```python
from build123d import *

# Parameters (mm, degrees)
RESSALTO_EXTRUS_O2_DEPTH      = 30
RESSALTO_EXTRUS_O3_DEPTH      = 3
RESSALTO_EXTRUS_O4_DEPTH      = 3
RESSALTO_EXTRUS_O4_DEPTH_BACK = 10


with BuildPart() as part:
    # Esboço2 → Ressalto-extrusão2 (new body)
    with BuildSketch(Plane(origin=(0, 0, 0), x_dir=(0, 0, -1), z_dir=(1, 0, 0))):
        with BuildLine():
            Line((2.90159992, -0.062465938), (-35.09840008, -0.062465938))
            Line((-35.09840008, -0.062465938), (-39.886084903, -0.062465938))
            ThreePointArc((-39.886084903, -0.062465938), (-45.202180234, 1.467638524), (-48.891439328, 5.589707975))
            ThreePointArc((-48.891439328, 5.589707975), (-52.096536948, 9.772081499), (-56.69840008, 12.338743681))
            ThreePointArc((-56.69840008, 12.338743681), (-59.373224015, 11.895603401), (-60.59840008, 9.476926077))
            Line((-60.59840008, 9.476926077), (-60.59840008, 20.976926077))
            ThreePointArc((-60.59840008, 20.976926077), (-59.719720424, 23.09824642), (-57.59840008, 23.976926077))
            Line((-57.59840008, 23.976926077), (25.40159992, 23.976926077))
            ThreePointArc((25.40159992, 23.976926077), (27.522920263, 23.09824642), (28.40159992, 20.976926077))
            Line((28.40159992, 20.976926077), (28.40159992, 9.476926077))
            ThreePointArc((28.40159992, 9.476926077), (27.176423855, 11.895603401), (24.50159992, 12.338743681))
            ThreePointArc((24.50159992, 12.338743681), (19.899736788, 9.772081499), (16.694639168, 5.589707975))
            ThreePointArc((16.694639168, 5.589707975), (13.005380073, 1.467638524), (7.689284743, -0.062465938))
            Line((7.689284743, -0.062465938), (2.90159992, -0.062465938))
        make_face()
    extrude(amount=RESSALTO_EXTRUS_O2_DEPTH)

    # Esboço3 → Ressalto-extrusão3 (add)
    with BuildSketch(Plane.ZY):
        with BuildLine():
            Line((60.59840008, 15.226926077), (60.59840008, 20.976926077))
            ThreePointArc((60.59840008, 20.976926077), (59.719720424, 23.09824642), (57.59840008, 23.976926077))
            Line((57.59840008, 23.976926077), (16.09840008, 23.976926077))
            Line((16.09840008, 23.976926077), (-25.40159992, 23.976926077))
            ThreePointArc((-25.40159992, 23.976926077), (-27.522920263, 23.09824642), (-28.40159992, 20.976926077))
            Line((-28.40159992, 20.976926077), (-28.40159992, 15.226926077))
            Line((-28.40159992, 15.226926077), (-28.40159992, -16.773073923))
            ThreePointArc((-28.40159992, -16.773073923), (-27.522920263, -18.894394267), (-25.40159992, -19.773073923))
            Line((-25.40159992, -19.773073923), (57.59840008, -19.773073923))
            ThreePointArc((57.59840008, -19.773073923), (59.719720424, -18.894394267), (60.59840008, -16.773073923))
            Line((60.59840008, -16.773073923), (60.59840008, 15.226926077))
        make_face()
    extrude(amount=RESSALTO_EXTRUS_O3_DEPTH)

    # Esboço4 → Ressalto-extrusão4 (add, two sides)
    with BuildSketch(Plane(origin=(30, 0, 0), x_dir=(0, 0, -1), z_dir=(1, 0, 0))) as ressalto_extrus_o4_sk:
        with BuildLine():
            Line((-16.09840008, 23.976926077), (25.40159992, 23.976926077))
            ThreePointArc((25.40159992, 23.976926077), (27.522920263, 23.09824642), (28.40159992, 20.976926077))
            Line((28.40159992, 20.976926077), (28.40159992, 15.226926077))
            Line((28.40159992, 15.226926077), (28.40159992, -16.773073923))
            ThreePointArc((28.40159992, -16.773073923), (27.522920263, -18.894394267), (25.40159992, -19.773073923))
            Line((25.40159992, -19.773073923), (-57.59840008, -19.773073923))
            ThreePointArc((-57.59840008, -19.773073923), (-59.719720424, -18.894394267), (-60.59840008, -16.773073923))
            Line((-60.59840008, -16.773073923), (-60.59840008, 15.226926077))
            Line((-60.59840008, 15.226926077), (-60.59840008, 20.976926077))
            ThreePointArc((-60.59840008, 20.976926077), (-59.719720424, 23.09824642), (-57.59840008, 23.976926077))
            Line((-57.59840008, 23.976926077), (-16.09840008, 23.976926077))
        make_face()
    extrude(amount=RESSALTO_EXTRUS_O4_DEPTH)
    extrude(ressalto_extrus_o4_sk.sketch, amount=-RESSALTO_EXTRUS_O4_DEPTH_BACK)


solid = part.part
```
For this review, take the finished solid that the model builds, in its own axes (mm). A direction names the side the tool comes from. Round coordinates to 2 decimals unless told otherwise and drop trailing zeros. Write each loop counter-clockwise with the first axis right and the second up, starting at its lowest first coordinate (ties: lowest second). Pieces come first, ordered by that corner, then holes. Notation, with made-up numbers: M 35,53.5 L 56,53.5 A30 ccw 56,86.5 Z; hole C 41,-18.5 d9. An arc over 180 degrees is marked long. One line per item, written item: value. Start each with the question number.
(1) We need section A-A (x = 16). Give the boundary of the cut face in (y, z), and give its area (3 significant figures).
(2) Machinability: for faces 1 (the flat face through (10, -0.062, 16)), 2 (the cylindrical face through (9.86, 1.51, -13.07)), 3 (the cylindrical face through (9.86, 9.821, -19.956)), 4 (the cylindrical face through (9.86, 1.43, 45.14)), which of the approach directions +Z, -Z, +X, -X, +Y, -Y give a long, thin tool a straight path to every point of the face, cutting with its end or side? Answer none if there is none.
(3) The part is to be moulded in two halves that separate along Z. For faces 5 (the cylindrical face through (9.86, 9.723, 52.04)), 6 (the cylindrical face through (-1.479, -18.871, -27.546)), 7 (the flat face through (15, 23.977, 17)), say which applies: released by +Z, released by -Z, zero draft, split by the parting line, or undercut.
(4) Wall thickness on line 1 (X direction, y = -15, z = -9.5); line 2 (Y direction, x = 11, z = 34.5); line 3 (Z direction, x = 14.5, y = 1): over which ranges is each line inside the solid? List them lowest first.
(5) We need section C-C (z = 14). Give the boundary of the cut face in (x, y).
(6) We need section D-D (y = 10.5). Give the boundary of the cut face in (x, z), and give its area (3 significant figures).
(7) Insertion check: pin 1 (12 mm diameter, centred on x = 10, z = 14.5, fed in from -Y). The pin has a flat end and moves straight along its axis. Give the tip position at first contact, or say it passes through.
(8) We need section B-B (y = -12). Give the boundary of the cut face in (x, z).
Result:
1. outline: M -0.06,-7.69 A10 ccw 5.59,-16.69 A13 cw 12.34,-24.5 A3 cw 9.48,-28.4 L 20.98,-28.4 A3 ccw 23.98,-25.4 L 23.98,57.6 A3 ccw 20.98,60.6 L 9.48,60.6 A3 cw 12.34,56.7 A13 cw 5.59,48.89 A10 ccw -0.06,39.89 Z
1. area: 1,860 mm²
2. face 1: +Z, -Z, -Y
2. face 2: -Z, -Y
2. face 3: -Y
2. face 4: +Z, -Y
3. face 5: undercut
3. face 6: released by -Z
3. face 7: zero draft
4. line 1: -3 to 0, 20 to 33
4. line 2: -0.06 to 23.98
4. line 3: -12.17 to 44.37
5. outline: M -3,-19.77 L 0,-19.77 L 0,-0.06 L 20,-0.06 L 20,-19.77 L 33,-19.77 L 33,23.98 L -3,23.98 Z
6. outline: M -3,-28.4 L 33,-28.4 L 33,60.6 L -3,60.6 Z; hole M 0,-28.22 L 20,-28.22 L 20,-20.82 L 0,-20.82 Z; hole M 0,53.02 L 20,53.02 L 20,60.42 L 0,60.42 Z
6. area: 2,910 mm²
7. pin 1: y = -0.06
8. outline: M -3,-28.4 L 0,-28.4 L 0,60.6 L -3,60.6 Z; M 20,-28.4 L 33,-28.4 L 33,60.6 L 20,60.6 Z
